The model under review builds one solid part; all positions refer to its coordinate system, in mm. A direction names the side the tool comes from. Round coordinates to 2 decimals unless told otherwise and drop trailing zeros. Loops run counter-clockwise (first coordinate to the right, second up) from the corner with the lowest first, then second, coordinate; pieces in that order, holes last. Notation, with made-up numbers: (61, -7) -> (111, -7) arc R20 cw to (111, 17) -> close; hole circle Ø7 at (-11.5, 76.5). An arc over 180 degrees is marked (long way). Return JSON: item names as keys, results as strings. Group by question number.
Autodesk Inventor part; units mm, degrees
ref_plane "YZ Plane" through (0, 0, 0) normal (1, 0, 0) x (0, 1, 0)
ref_plane "XZ Plane" through (0, 0, 0) normal (0, 1, 0) x (-1, 0, 0)
ref_plane "XY Plane" through (0, 0, 0) normal (0, 0, 1) x (1, 0, 0)
sketch "Sketch1" plane through (0, 0, 0) normal (0, 0, 1) x (1, 0, 0)
  line L0 (-3.5739, 7.4603) -> (-3.5739, -5.2397)
  line L1 (-3.5739, -5.2397) -> (109.9387, -5.2397)
  line L2 (109.9387, -5.2397) -> (109.9387, 1.1103)
  line L3 (109.9387, 1.1103) -> (0.3885, 1.1103)
  line L4 (0.3885, 1.1103) -> (0.3885, 7.4603)
  line L5 (0.3885, 7.4603) -> (-3.5739, 7.4603)
  line L6 (-3.5739, 7.4603) -> (-3.5739, 9.8416)
  line L7 (-3.5739, 9.8416) -> (113.4449, 9.8416)
  point P0 (0, 0)
  dimension "d0" = 3.9624
  dimension "d1" = 113.5126
  dimension "d2" = 6.35
  dimension "d3" = 12.7
  dimension "d4" = 2.3813
revolve "Revolution1" add sketch "Sketch1" angle 360 about axis through (-3.5739, 9.8416, 0) along (1, 0, 0)
fillet "Fillet1" radius 6.35 1 edges at (109.9387, 24.9228, 0)
fillet "Fillet2" radius 6.35 1 edges at (-3.5739, 24.9228, 0)
properties part number "handle bar" material "Rubber"
1. We need section B-B, the plane x = 36. Write out the cut boundary in (y, z).
2. Draft analysis for pull direction Z (two halves, no side actions). For faces 1 (the face through (0.388, 8, 2)), 2 (the face through (53.888, 13.111, 14.723)), 3 (the face through (-3.574, 8, 2)), state which applies: pulls with the +Z half, pulls with the -Z half, needs draft (parallel to the pull), parting line crosses it, or undercut.
3. Tool access review of faces 4 (the face through (-1.62, 12.22, 0.1)), 5 (the face through (54.397, 1.513, 2.623)): name each direction out of +Z, -Z, +X, -X, +Y, -Y from which nothing blocks a thin tool from reaching the whole face with its end or side.
4. Wall thickness on line 1 (Z direction, x = 66, y = 4); line 2 (Y direction, x = -2.2, z = 0); line 3 (Y direction, x = 58, z = 0): over which ranges is each line inside the solid? List them lowest first.
5. For P1, Ø4, axis at x = 79.5, y = -2, coming from the +Z side; P2, Ø7.5, axis at y = 9.84, z = 0, coming from the -X side; P3, Ø6, axis at x = 82.5, z = -5.5, coming from the -Y side; P4, Ø6, axis at y = 21.5, z = -10, coming from the -X side, all flat-tipped, find the tip position at first contact; note any pin that passes through.
Check sheet entries:
{
 "1": {"outline": "circle Ø30.16 at (9.84, 0); hole circle Ø17.46 at (9.84, 0)"},
 "2": {"face 1": "undercut", "face 2": "parting line crosses it", "face 3": "needs draft"},
 "3": {"face 4": "+X, -X", "face 5": "+X"},
 "4": {"line 1": "z = -13.9 to -6.49, 6.49 to 13.9", "line 2": "y = -2.83 to 7.46, 12.22 to 22.52", "line 3": "y = -5.24 to 1.11, 18.57 to 24.92"},
 "5": {"P1": "stops at z = 11.43", "P2": "stops at x = -3.57", "P3": "stops at y = -5.03", "P4": "stops at x = -2.44"}
}
